CAD build for the part. Positions are in the model's coordinates, mm. A direction names the side the tool comes from. Give positions to 0.01 mm unless a question says otherwise; leave off trailing zeros. Write each loop counter-clockwise with the first axis right and the second up, starting at its lowest first coordinate (ties: lowest second). Pieces come first, ordered by that corner, then holes. Notation, with made-up numbers: (71, 44.5) - (91, 44.5) arc R22 ccw to (91, 58.5) - close; hole circle Ø1 at (69.25, 5). An arc over 180 degrees is marked (long way). Answer as a JSON object with one key per item and string values.
from build123d import *

# Parameters (mm, degrees)
BOSS_EXTRUDE1_DEPTH = 30
CUT_EXTRUDE1_REACH  = 38.851
SKETCH5_R           = 4
BOSS_EXTRUDE2_START = 3
SKETCH6_R           = 5.5
SKETCH6_R_2         = 4
BOSS_EXTRUDE2_DEPTH = 3
SKETCH7_R           = 5.5
SKETCH7_R_2         = 4
BOSS_EXTRUDE3_DEPTH = 3
SKETCH8_R           = 2
CUT_EXTRUDE2_DEPTH  = 6
SKETCH9_R           = 1.7
CUT_EXTRUDE3_DEPTH  = 10


with BuildPart() as part:
    # Sketch1 → Boss-Extrude1 (new body)
    with BuildSketch(Plane.XY):
        with BuildLine():
            Line((-9.38083152, -9), (-17, -9))
            Line((-17, -9), (-17, 9))
            Line((-17, 9), (17, 9))
            Line((17, 9), (17, -9))
            Line((17, -9), (9.38083152, -9))
            ThreePointArc((9.38083152, -9), (0, -13), (-9.38083152, -9))
        make_face()
    extrude(amount=BOSS_EXTRUDE1_DEPTH)

    # Sketch5 → Cut-Extrude1 (cut, up to next)
    with BuildSketch(Plane.XY.offset(30), mode=Mode.PRIVATE) as cut_extrude1_sk1:
        with Locations((0, -2)):
            Circle(SKETCH5_R)
    cut_extrude1_tool1 = extrude(cut_extrude1_sk1.sketch, amount=-CUT_EXTRUDE1_REACH, mode=Mode.PRIVATE) & part.part
    add(cut_extrude1_tool1.solids().sort_by_distance((0, -2, 30))[0], mode=Mode.SUBTRACT)

    # Sketch6 → Boss-Extrude2 (add)
    with BuildSketch(Plane.XY.offset(30).offset(BOSS_EXTRUDE2_START)):
        with Locations((0, -2)):
            Circle(SKETCH6_R)
        with Locations((0, -2)):
            Circle(SKETCH6_R_2, mode=Mode.SUBTRACT)
    extrude(amount=-BOSS_EXTRUDE2_DEPTH)

    # Sketch7 → Boss-Extrude3 (add)
    with BuildSketch(Plane(origin=(0, 0, 0), x_dir=(-1, 0, 0), z_dir=(0, 0, -1))):
        with Locations(Location((0, -2, 0), (0, 0, 180))):
            Circle(SKETCH7_R)
        with Locations(Location((0, -2, 0), (0, 0, 180))):
            Circle(SKETCH7_R_2, mode=Mode.SUBTRACT)
    extrude(amount=BOSS_EXTRUDE3_DEPTH)

    # Sketch8 → Cut-Extrude2 (cut)
    with BuildSketch(Plane(origin=(0, 9, 0), x_dir=(1, 0, 0), z_dir=(0, 1, 0))):
        with Locations(Location((-12, -6, 0), (0, 0, 180))):
            Circle(SKETCH8_R)
        with Locations((-12, -24)):
            Circle(SKETCH8_R)
        with Locations(Location((12, -24, 0), (0, 0, 180))):
            Circle(SKETCH8_R)
        with Locations((12, -6)):
            Circle(SKETCH8_R)
    extrude(amount=-CUT_EXTRUDE2_DEPTH, mode=Mode.SUBTRACT)

    # Sketch9 → Cut-Extrude3 (cut)
    with BuildSketch(Plane.XZ.offset(9)):
        with Locations(Location((-12, 27, 0), (0, 0, 270))):
            Circle(SKETCH9_R)
        with Locations(Location((-12, 3, 0), (0, 0, 90))):
            Circle(SKETCH9_R)
        with Locations(Location((12, 3, 0), (0, 0, 270))):
            Circle(SKETCH9_R)
        with Locations(Location((12, 27, 0), (0, 0, 90))):
            Circle(SKETCH9_R)
    extrude(amount=-CUT_EXTRUDE3_DEPTH, mode=Mode.SUBTRACT)


solid = part.part
Item 1: Which spindle directions (+Z, -Z, +X, -X, +Y, -Y) get a long thin tool onto all of the face, cutting with end or side? Do faces 1 (the cylindrical face through (-4.4, -5.3, 31.5)), 2 (the flat face through (12, 1, 27)), 3 (the flat face through (13, -9, 15)). Say none if no direction does.
Entries:
{"face 1": "+Z", "face 2": "-Y", "face 3": "+Z, -Z, +X, -Y"}
Item 2: Flat gauge pins, fed straight in: P1, Ø2.5, axis at x = -12, z = 24, coming from the -Y side; P2, Ø1.7, axis at x = -12.5, z = 2.5, coming from the -Y side; P3, Ø1.2, axis at x = 12, z = 23, coming from the +Y side. Where does each tip first touch, or does it go through?
Entries:
{"P1": "y = -9", "P2": "y = 1", "P3": "y = 3"}
Item 3: Probe line 1 (Z direction, x = -12, y = 5.8); line 2 (Z direction, x = -13.5, y = -7); line 3 (Z direction, x = -8.5, y = -8.5). List the from-to ranges inside material, lowest first. Write a range as from..to.
Entries:
{"line 1": "0..4, 8..22, 26..30", "line 2": "0..2.2, 3.8..26.2, 27.8..30", "line 3": "0..30"}
Item 4: Cut at C-C (z = 3). Give the cut face in (x, y), and give its area (3 significant figures).
Entries:
{"outline": "(-17, -9) - (-13.7, -9) - (-13.7, 1) - (-10.3, 1) - (-10.3, -9) - (-9.38, -9) arc R13 ccw to (9.38, -9) - (10.3, -9) - (10.3, 1) - (13.7, 1) - (13.7, -9) - (17, -9) - (17, 9) - (-17, 9) - close; hole circle Ø8 at (0, -2)", "area": "546 mm2"}
Item 5: Cut at A-A (x = 0). Give the cut face in (y, z).
Entries:
{"outline": "(-13, 0) - (-7.5, 0) - (-7.5, -3) - (-6, -3) - (-6, 33) - (-7.5, 33) - (-7.5, 30) - (-13, 30) - close; (2, -3) - (3.5, -3) - (3.5, 0) - (9, 0) - (9, 30) - (3.5, 30) - (3.5, 33) - (2, 33) - close"}
Item 6: Cut at B-B (y = 7). Give the cut face in (x, z).
Entries:
{"outline": "(-17, 0) - (17, 0) - (17, 30) - (-17, 30) - close; hole circle Ø4 at (-12, 6); hole circle Ø4 at (-12, 24); hole circle Ø4 at (12, 6); hole circle Ø4 at (12, 24)"}
Item 7: Cut at D-D (y = -2.5). Give the cut face in (x, z).
Entries:
{"outline": "(-17, 0) - (-5.48, 0) - (-5.48, -3) - (-3.97, -3) - (-3.97, 33) - (-5.48, 33) - (-5.48, 30) - (-17, 30) - close; (3.97, -3) - (5.48, -3) - (5.48, 0) - (17, 0) - (17, 30) - (5.48, 30) - (5.48, 33) - (3.97, 33) - close; hole circle Ø3.4 at (-12, 3); hole circle Ø3.4 at (-12, 27); hole circle Ø3.4 at (12, 3); hole circle Ø3.4 at (12, 27)"}
Item 8: Mould opens along Z. For faces 4 (the flat face through (-13, -9, 15)), 5 (the flat face through (-12, 3, 6)), 6 (the flat face through (4, 3, 30)) say: +Z half, -Z half, draft (parallel to the pull), parting line (faces both ways), or undercut.
Entries:
{"face 4": "draft", "face 5": "undercut", "face 6": "+Z half"}
